from build123d import *

# Parameters (mm, degrees)
F0_R     = 3.2
F1_DEPTH = 19
F2_DEPTH = 5


with BuildPart() as f1:
    # F0 (on Top) → F1 (new body)
    with BuildSketch(Plane.XY):
        with BuildLine():
            Line((-16.083093, 46.314633), (-77.51673, 46.314633))
            ThreePointArc((-77.51673, 46.314633), (-83.608573, 24.668741), (-76.936605, 3.194569))
            Line((-76.936605, 3.194569), (-4.737342, 3.194569))
            ThreePointArc((-4.737342, 3.194569), (-6.8374, 25.694681), (-16.083093, 46.314633))
        make_face()
        with Locations((-73.675402, 8.108267)):
            Circle(F0_R, mode=Mode.SUBTRACT)
        with BuildLine():
            ThreePointArc((-77.366346, 40.272824), (-75.521531, 42.415285), (-72.809609, 43.214634))
            Line((-72.809609, 43.214634), (-20.607641, 43.214634))
            ThreePointArc((-20.607641, 43.214634), (-18.091299, 42.535285), (-16.258748, 40.681845))
            ThreePointArc((-16.258748, 40.681845), (-10.294291, 26.562128), (-7.746958, 11.447491))
            ThreePointArc((-7.746958, 11.447491), (-9.116704, 7.749617), (-12.740557, 6.194569))
            Line((-12.740557, 6.194569), (-63.759234, 6.194569))
            ThreePointArc((-63.759234, 6.194569), (-66.72323, 7.167817), (-68.533345, 9.708678))
            ThreePointArc((-68.533345, 9.708678), (-70.739665, 12.623078), (-74.298513, 13.457453))
            ThreePointArc((-74.298513, 13.457453), (-77.779678, 14.352671), (-79.760766, 17.351873))
            ThreePointArc((-79.760766, 17.351873), (-80.414005, 29.005654), (-77.366346, 40.272824))
        make_face(mode=Mode.SUBTRACT)
    extrude(amount=F1_DEPTH)

    # F0 (on Top) → F2 (join)
    with BuildSketch(Plane.XY):
        with BuildLine():
            Line((-20.607641, 43.214634), (-72.809609, 43.214634))
            ThreePointArc((-72.809609, 43.214634), (-75.521531, 42.415285), (-77.366346, 40.272824))
            ThreePointArc((-77.366346, 40.272824), (-80.414005, 29.005654), (-79.760766, 17.351873))
            ThreePointArc((-79.760766, 17.351873), (-77.779678, 14.352671), (-74.298513, 13.457453))
            ThreePointArc((-74.298513, 13.457453), (-70.739665, 12.623078), (-68.533345, 9.708678))
            ThreePointArc((-68.533345, 9.708678), (-66.72323, 7.167817), (-63.759234, 6.194569))
            Line((-63.759234, 6.194569), (-12.740557, 6.194569))
            ThreePointArc((-12.740557, 6.194569), (-9.116704, 7.749617), (-7.746958, 11.447491))
            ThreePointArc((-7.746958, 11.447491), (-10.294291, 26.562128), (-16.258748, 40.681845))
            ThreePointArc((-16.258748, 40.681845), (-18.091299, 42.535285), (-20.607641, 43.214634))
        make_face()
    extrude(amount=F2_DEPTH)


solid = f1.part
Could you check a few things on this model? Use its own coordinates, in mm. A direction names the side the tool comes from. Round coordinates to 2 decimals unless told otherwise and drop trailing zeros. Order: outer loops, then holes, each group sorted by start corner. A loop starts at its lowest first (then second) coordinate and runs counter-clockwise, first axis right, second up.
(1) Imagine slicing it at D-D (x = -28.5). Write out the boundary of the cut face in (y, z).
Response values:
outline: (3.19, 0) - (46.31, 0) - (46.31, 19) - (43.21, 19) - (43.21, 5) - (6.19, 5) - (6.19, 19) - (3.19, 19) - close
(2) If we mould it in two halves opening along X, with no side actions, what happens to faces 3 (the cylindrical face through (-83.61, 24.99, 9.37)), 4 (the cylindrical face through (-66.687, 7.142, 11.902)), 5 (the cylindrical face through (-9.08, 7.79, 11.9)), 6 (the flat face through (-41, 3.195, 9))? For each: released by +X, released by -X, zero draft, split by the parting line, or undercut.
Response values:
face 3: released by -X
face 4: undercut
face 5: undercut
face 6: zero draft
(3) Imagine slicing it at B-B (x = -75.5). Write out the boundary of the cut face in (y, z), plus the area to 3 significant figures.
Response values:
outline: (3.19, 0) - (5.48, 0) - (5.48, 19) - (3.19, 19) - close; (10.74, 0) - (46.31, 0) - (46.31, 19) - (42.43, 19) - (42.43, 5) - (13.46, 5) - (13.46, 19) - (10.74, 19) - close
area: 314 mm2
(4) Please list where these lines run through material, in increasing order: line 1 along Y through (x, z) = (-54.5, 12.75); line 2 along Y through (x, z) = (-71.5, 16); line 3 along X through (y, z) = (7, 14.75).
Response values:
line 1: y = 3.19 to 6.19, 43.21 to 46.31
line 2: y = 3.19 to 5.76, 10.46 to 13.03, 43.21 to 46.31
line 3: x = -79.18 to -76.68, -70.67 to -66.48, -10.02 to -4.57
(5) Which directions (+Z, -Z, +X, -X, +Y, -Y) give clear straight access to the entire face, cutting with the end or side of a thin tool? Please do faces 1 (the flat face through (-45, 25, 0)), 2 (the flat face through (-45, 25, 5)).
Response values:
face 1: -Z, +X, -X, +Y, -Y
face 2: +Z
(6) I'm going to push flat-ended pins straight in: pin 1 (6 mm diameter, centred on y = 16.5, z = 16.5, fed in from -X); pin 2 (8 mm diameter, centred on y = 28, z = 16.5, fed in from +X). Where does each tip first touch, or does it pass through?
Response values:
pin 1: stops at x = -83.2
pin 2: stops at x = -6.41
(7) Imagine slicing it at A-A (z = 6.75). Write out the boundary of the cut face in (x, y), plus the area to 3 significant figures.
Response values:
outline: (-77.52, 46.31) arc R39.61 ccw to (-76.94, 3.19) - (-4.74, 3.19) arc R69.11 ccw to (-16.08, 46.31) - close; hole (-79.76, 17.35) arc R5 ccw to (-74.3, 13.46) arc R5.39 cw to (-68.53, 9.71) arc R5 ccw to (-63.76, 6.19) - (-12.74, 6.19) arc R5 ccw to (-7.75, 11.45) arc R66.01 ccw to (-16.26, 40.68) arc R5 ccw to (-20.61, 43.21) - (-72.81, 43.21) arc R5 ccw to (-77.37, 40.27) arc R36.61 ccw to start; hole circle Ø6.4 at (-73.68, 8.11)
area: 694 mm2
(8) Imagine slicing it at C-C (y = 37). Write out the boundary of the cut face in (x, z).
Response values:
outline: (-81.81, 0) - (-10.89, 0) - (-10.89, 19) - (-14.32, 19) - (-14.32, 5) - (-78.66, 5) - (-78.66, 19) - (-81.81, 19) - close
